Geometry check sheet. Reference: the model listing, model coordinates, mm. A direction names the side the tool comes from. Round coordinates to 2 decimals unless told otherwise and drop trailing zeros. Write each loop counter-clockwise with the first axis right and the second up, starting at its lowest first coordinate (ties: lowest second). Pieces come first, ordered by that corner, then holes. Notation, with made-up numbers: (27.5, 62) -> (46.5, 62) arc R22 cw to (46.5, 77) -> close; hole circle Ø5 at (-15.5, -8.5). An arc over 180 degrees is marked (long way). Use a Markdown table: item, result.
```python
from build123d import *

# Parameters (mm, degrees)
F1_DEPTH = 7.5


with BuildPart() as f1:
    # F0 (on Top) → F1 (new body)
    with BuildSketch(Plane.XY):
        with BuildLine():
            ThreePointArc((-22.4461433303, 26.7502719537), (-17.46, 30.2416071002), (-11.9433434049, 32.8140663178))
            Line((-11.9433434049, 32.8140663178), (-13.680805733, 37.5877048314))
            ThreePointArc((-13.680805733, 37.5877048314), (-20, 34.6410161514), (-25.7115043875, 30.6417777248))
            Line((-25.7115043875, 30.6417777248), (-22.4461433303, 26.7502719537))
        make_face()
        with BuildLine():
            ThreePointArc((-22.4461433303, -26.7502719537), (-34.92, 0), (-22.4461433303, 26.7502719537))
            Line((-22.4461433303, 26.7502719537), (-25.7115043875, 30.6417777248))
            ThreePointArc((-25.7115043875, 30.6417777248), (-40, 0), (-25.7115043875, -30.6417777248))
            Line((-25.7115043875, -30.6417777248), (-22.4461433303, -26.7502719537))
        make_face()
        with BuildLine():
            ThreePointArc((-11.9433434049, 32.8140663178), (17.46, 30.2416071002), (34.3894867352, 6.0637943641))
            Line((34.3894867352, 6.0637943641), (39.3923101205, 6.9459271067))
            ThreePointArc((39.3923101205, 6.9459271067), (20, 34.6410161514), (-13.680805733, 37.5877048314))
            Line((-13.680805733, 37.5877048314), (-11.9433434049, 32.8140663178))
        make_face()
        with BuildLine():
            Line((39.3923101205, 6.9459271067), (34.3894867352, 6.0637943641))
            ThreePointArc((34.3894867352, 6.0637943641), (34.7871188574, 3.0434785367), (34.92, 0))
            ThreePointArc((34.92, 0), (34.7871188574, -3.0434785367), (34.3894867352, -6.0637943641))
            Line((34.3894867352, -6.0637943641), (39.3923101205, -6.9459271067))
            ThreePointArc((39.3923101205, -6.9459271067), (39.8477879237, -3.4862297099), (40, 0))
            ThreePointArc((40, 0), (39.8477879237, 3.4862297099), (39.3923101205, 6.9459271067))
        make_face()
        with BuildLine():
            Line((34.3894867352, 6.0637943641), (15.8357086684, 2.7922626969))
            ThreePointArc((15.8357086684, 2.7922626969), (16.0188107453, 1.4014643434), (16.08, 0))
            ThreePointArc((16.08, 0), (16.0188107453, -1.4014643434), (15.8357086684, -2.7922626969))
            Line((15.8357086684, -2.7922626969), (34.3894867352, -6.0637943641))
            ThreePointArc((34.3894867352, -6.0637943641), (34.7871188574, -3.0434785367), (34.92, 0))
            ThreePointArc((34.92, 0), (34.7871188574, 3.0434785367), (34.3894867352, 6.0637943641))
        make_face()
        with BuildLine():
            ThreePointArc((10.8328852831, 1.9101299543), (10.958141679, 0.9587131702), (11, 0))
            ThreePointArc((11, 0), (10.958141679, -0.9587131702), (10.8328852831, -1.9101299543))
            Line((10.8328852831, -1.9101299543), (15.8357086684, -2.7922626969))
            ThreePointArc((15.8357086684, -2.7922626969), (16.0188107453, -1.4014643434), (16.08, 0))
            ThreePointArc((16.08, 0), (16.0188107453, 1.4014643434), (15.8357086684, 2.7922626969))
            Line((15.8357086684, 2.7922626969), (10.8328852831, 1.9101299543))
        make_face()
        with BuildLine():
            ThreePointArc((-3.7622215766, 10.3366188286), (5.5, 9.5262794416), (10.8328852831, 1.9101299543))
            Line((10.8328852831, 1.9101299543), (15.8357086684, 2.7922626969))
            ThreePointArc((15.8357086684, 2.7922626969), (8.04, 13.9256884929), (-5.4996839047, 15.1102573422))
            Line((-5.4996839047, 15.1102573422), (-3.7622215766, 10.3366188286))
        make_face()
        with BuildLine():
            ThreePointArc((-7.0706637066, 8.4264888743), (-5.5, 9.5262794416), (-3.7622215766, 10.3366188286))
            Line((-3.7622215766, 10.3366188286), (-5.4996839047, 15.1102573422))
            ThreePointArc((-5.4996839047, 15.1102573422), (-8.04, 13.9256884929), (-10.3360247638, 12.3179946454))
            Line((-10.3360247638, 12.3179946454), (-7.0706637066, 8.4264888743))
        make_face()
        with BuildLine():
            ThreePointArc((-10.3360247638, 12.3179946454), (-8.04, 13.9256884929), (-5.4996839047, 15.1102573422))
            Line((-5.4996839047, 15.1102573422), (-11.9433434049, 32.8140663178))
            ThreePointArc((-11.9433434049, 32.8140663178), (-17.46, 30.2416071002), (-22.4461433303, 26.7502719537))
            Line((-22.4461433303, 26.7502719537), (-10.3360247638, 12.3179946454))
        make_face()
        with BuildLine():
            ThreePointArc((-7.0706637066, -8.4264888743), (-11, 0), (-7.0706637066, 8.4264888743))
            Line((-7.0706637066, 8.4264888743), (-10.3360247638, 12.3179946454))
            ThreePointArc((-10.3360247638, 12.3179946454), (-16.08, 0), (-10.3360247638, -12.3179946454))
            Line((-10.3360247638, -12.3179946454), (-7.0706637066, -8.4264888743))
        make_face()
        with BuildLine():
            Line((-5.4996839047, -15.1102573422), (-3.7622215766, -10.3366188286))
            ThreePointArc((-3.7622215766, -10.3366188286), (-5.5, -9.5262794416), (-7.0706637066, -8.4264888743))
            Line((-7.0706637066, -8.4264888743), (-10.3360247638, -12.3179946454))
            ThreePointArc((-10.3360247638, -12.3179946454), (-8.04, -13.9256884929), (-5.4996839047, -15.1102573422))
        make_face()
        with BuildLine():
            Line((15.8357086684, -2.7922626969), (10.8328852831, -1.9101299543))
            ThreePointArc((10.8328852831, -1.9101299543), (5.5, -9.5262794416), (-3.7622215766, -10.3366188286))
            Line((-3.7622215766, -10.3366188286), (-5.4996839047, -15.1102573422))
            ThreePointArc((-5.4996839047, -15.1102573422), (8.04, -13.9256884929), (15.8357086684, -2.7922626969))
        make_face()
        with BuildLine():
            Line((-11.9433434049, -32.8140663178), (-5.4996839047, -15.1102573422))
            ThreePointArc((-5.4996839047, -15.1102573422), (-8.04, -13.9256884929), (-10.3360247638, -12.3179946454))
            Line((-10.3360247638, -12.3179946454), (-22.4461433303, -26.7502719537))
            ThreePointArc((-22.4461433303, -26.7502719537), (-17.46, -30.2416071002), (-11.9433434049, -32.8140663178))
        make_face()
        with BuildLine():
            Line((-13.680805733, -37.5877048314), (-11.9433434049, -32.8140663178))
            ThreePointArc((-11.9433434049, -32.8140663178), (-17.46, -30.2416071002), (-22.4461433303, -26.7502719537))
            Line((-22.4461433303, -26.7502719537), (-25.7115043875, -30.6417777248))
            ThreePointArc((-25.7115043875, -30.6417777248), (-20, -34.6410161514), (-13.680805733, -37.5877048314))
        make_face()
        with BuildLine():
            Line((39.3923101205, -6.9459271067), (34.3894867352, -6.0637943641))
            ThreePointArc((34.3894867352, -6.0637943641), (17.46, -30.2416071002), (-11.9433434049, -32.8140663178))
            Line((-11.9433434049, -32.8140663178), (-13.680805733, -37.5877048314))
            ThreePointArc((-13.680805733, -37.5877048314), (20, -34.6410161514), (39.3923101205, -6.9459271067))
        make_face()
    extrude(amount=F1_DEPTH)


solid = f1.part
```
(1) Access from +Z, -Z, +X, -X, +Y, -Y to the whole of each face (thin tool, end or side, straight path). Record for faces 3 (the face through (-16.306, -19.433, 3.698)), 4 (the face through (8, -8, 0)).
A:
| item | result |
|---|---|
| face 3 | +Z, -Z |
| face 4 | -Z, +X, -X, +Y, -Y |
(2) Section check C-C on x = 31.5. Record the cut outline in (y, z).
A:
| item | result |
|---|---|
| outline | (-24.65, 0) -> (-15.07, 0) -> (-15.07, 7.5) -> (-24.65, 7.5) -> close; (-5.55, 0) -> (5.55, 0) -> (5.55, 7.5) -> (-5.55, 7.5) -> close; (15.07, 0) -> (24.65, 0) -> (24.65, 7.5) -> (15.07, 7.5) -> close |
(3) Thickness scan on line 1 (Y direction, x = 14.5, z = 7.25); line 2 (Y direction, x = 22, z = 1.75); line 3 (X direction, y = -26, z = 7). Record the ranges inside material, lowest first.
A:
| item | result |
|---|---|
| line 1 | y = -37.28 to -31.77, -6.95 to 6.95, 31.77 to 37.28 |
| line 2 | y = -33.41 to -27.12, -3.88 to 3.88, 27.12 to 33.41 |
| line 3 | x = -30.4 to -23.31, -21.82 to -9.46, 23.31 to 30.4 |
(4) Release check for a two-part mould opening along Y. For faces 1 (the face through (-8.676, 23.838, 3.698)), 2 (the face through (8, -8, 7.5)) record: +Y half, -Y half, draft (parallel to the pull), parting line (faces both ways), or undercut.
A:
| item | result |
|---|---|
| face 1 | undercut |
| face 2 | draft |
(5) Gauge pin test, flat ends, axial feed: pin 1 Ø1 at (x, z) = (-30.5, 6) entering from +Y; pin 2 Ø4 at (y, z) = (5, 4) entering from -X; pin 3 Ø2 at (x, y) = (27.5, -16.5) entering from -Z; pin 4 Ø1 at (x, z) = (-17, 1) entering from +Y. Record the tip position at first contact, or that the pin passes through.
A:
| item | result |
|---|---|
| pin 1 | stops at y = 26.46 |
| pin 2 | stops at x = -39.89 |
| pin 3 | passes through |
| pin 4 | stops at y = 36.44 |
(6) Section check D-D on y = 4. Record the cut outline in (x, z).
A:
| item | result |
|---|---|
| outline | (-39.8, 0) -> (-34.69, 0) -> (-34.69, 7.5) -> (-39.8, 7.5) -> close; (-15.57, 0) -> (-10.25, 0) -> (-10.25, 7.5) -> (-15.57, 7.5) -> close; (10.25, 0) -> (15.57, 0) -> (15.57, 7.5) -> (10.25, 7.5) -> close; (22.69, 0) -> (39.8, 0) -> (39.8, 7.5) -> (22.69, 7.5) -> close |
(7) Section check B-B on y = -24.5. Record the cut outline in (x, z).
A:
| item | result |
|---|---|
| outline | (-31.62, 0) -> (-24.88, 0) -> (-24.88, 7.5) -> (-31.62, 7.5) -> close; (-20.56, 0) -> (-8.92, 0) -> (-8.92, 7.5) -> (-20.56, 7.5) -> close; (24.88, 0) -> (31.62, 0) -> (31.62, 7.5) -> (24.88, 7.5) -> close |
(8) Section check A-A on z = 4. Record the cut outline in (x, y), plus the area to 3 significant figures.
A:
| item | result |
|---|---|
| outline | circle Ø80 at (0, 0); hole (-22.45, -26.75) -> (-10.34, -12.32) arc R16.08 cw to (-10.34, 12.32) -> (-22.45, 26.75) arc R34.92 ccw to start; hole (-11.94, -32.81) arc R34.92 ccw to (34.39, -6.06) -> (15.84, -2.79) arc R16.08 cw to (-5.5, -15.11) -> close; hole (-11.94, 32.81) -> (-5.5, 15.11) arc R16.08 cw to (15.84, 2.79) -> (34.39, 6.06) arc R34.92 ccw to start; hole circle Ø22 at (0, 0) |
| area | 2,130 mm2 |
